CAD build for the part. Positions are in the model's coordinates, mm. A direction names the side the tool comes from. Round coordinates to 2 decimals unless told otherwise and drop trailing zeros. Answer as a JSON object with one key per item and string values.
```python
from build123d import *

# Parameters (mm, degrees)
F0_W          = 137.9242166877
F0_H          = 54.1928205639
F1_DEPTH      = 109.22
F1_TAPER      = -3
F2_T          = -5.08
F3_R          = 15.9007904293
F4_DEPTH      = 38.1
F4_TAPER      = -1
F5_T          = 2.54
F5_T3_DEPTH   = 109.5056366308
F5_T5_DEPTH   = 133.3627366899
F5_T7_DEPTH   = 109.5056366308
F5_T9_DEPTH   = 49.6313405661
F5_T11_DEPTH  = 109.5056366308
F5_T13_DEPTH  = 109.5056366308
F6_R          = 10.3601813923
F7_DEPTH      = 28.194
F7_DEPTH_BACK = 25.4


# Not quite as in the source:
# - a shell that OpenCascade refuses in one call is made with other operations: the cavity is built on its own and cut out


with BuildPart() as f1:
    # F0 (on Top) → F1 (new body)
    with BuildSketch(Plane.XY):
        with Locations((1.1629350483, -2.7910461649)):
            Rectangle(F0_W, F0_H)
    extrude(amount=F1_DEPTH, taper=F1_TAPER)

    # F2
    f2_openings = [f1.faces().sort_by_distance(p)[0] for p in [
        (1.162935, -2.791046, 109.22),
    ]]
    offset(amount=F2_T, openings=f2_openings)

    # F3 (on face) → F4 (join)
    with BuildSketch(Plane(origin=(0, -29.8055931401, -1.5620449467), x_dir=(1, 0, 0), z_dir=(0, -0.9986295348, -0.0523359562))):
        with Locations((0, 55.6432977319)):
            Circle(F3_R)
    extrude(amount=F4_DEPTH, taper=F4_TAPER)

    # F5: shell of thickness 2.54, made by hand


with BuildPart() as f5_core1:
    # F5_t2: copy of F1
    add(f1.part)

    # the walls: a layer under each face that stays
    f5_faces = [f5_core1.faces().sort_by_distance(p)[0] for p in [
        (1.1629350483, 27.1673529437, 54.61),
        (1.1629350483, -2.7910461649, 0),
        (-70.6611621221, -2.7910461649, 54.61),
        (72.0872036906, 9.6217245219, 109.22),
        (72.9870322188, -2.7910461649, 54.61),
        (-45.4478013646, -30.8414527224, 18.2033333333),
        (1.1629350483, -27.7955895152, 57.15),
        (68.0331764605, -2.7910461649, 57.15),
        (1.1629350483, 22.2134971854, 57.15),
        (-65.7073063639, -2.7910461649, 57.15),
        (-16.2333094162, -51.7416309725, 53.0079956131),
        (1.1629350483, -2.7910461649, 5.08),
    ]]
    thicken(f5_faces, amount=-F5_T, mode=Mode.SUBTRACT)

    # F5_s4 → F5_t3 (cut)
    with BuildSketch(Plane(origin=(-0.3725269372, -0.3725269372, 7.1082374087), x_dir=(0.7071067812, -0.7071067812, 0), z_dir=(-0.0522644277, -0.0522644277, 0.9972646886))):
        Polygon((-26.8076320701, -61.6755807303), (-25.0140422716, -63.5100601973), (-26.8076320701, -65.2987439692), (-28.6012218685, -63.5100601973), align=None)
    extrude(amount=F5_T3_DEPTH, mode=Mode.SUBTRACT)

    # F5_s6 → F5_t5 (cut)
    with BuildSketch(Plane.YZ.offset(-65.5184332966)):
        Polygon((-25.0413512578, 5.1067293333), (-27.6032354663, 4.9470666711), (-27.4770864474, 2.54), (-25.066716448, 2.54), align=None)
        Polygon((19.4592589279, 5.1067293333), (22.0211431364, 4.9470666711), (21.8949941176, 2.54), (19.4846241181, 2.54), align=None)
    extrude(amount=F5_T5_DEPTH, mode=Mode.SUBTRACT)

    # F5_s8 → F5_t7 (cut)
    with BuildSketch(Plane(origin=(0.3788802151, -0.3788802151, 7.229465173), x_dir=(0.7071067812, 0.7071067812, 0), z_dir=(0.0522644277, -0.0522644277, 0.9972646886))):
        Polygon((28.4522705876, -63.3157206494), (26.6586807892, -65.1502001164), (28.4522705876, -66.9388838882), (30.245860386, -65.1502001164), align=None)
    extrude(amount=F5_T7_DEPTH, mode=Mode.SUBTRACT)

    # F5_s10 → F5_t9 (cut)
    with BuildSketch(Plane.XZ.offset(-22.0246241181)):
        Polygon((65.2789382031, 5.1067293333), (67.8408224115, 4.9470666711), (67.7146733927, 2.54), (65.3043033933, 2.54), align=None)
        Polygon((-62.9530681064, 5.1067293333), (-65.5149523149, 4.9470666711), (-65.388803296, 2.54), (-62.9784332966, 2.54), align=None)
    extrude(amount=F5_T9_DEPTH, mode=Mode.SUBTRACT)

    # F5_s12 → F5_t11 (cut)
    with BuildSketch(Plane(origin=(6.0868817641, 6.0868817641, 116.1446229433), x_dir=(0.7071067812, -0.7071067812, 0), z_dir=(-0.0522644277, -0.0522644277, -0.9972646886))):
        Polygon((32.3994059273, -59.3793819539), (34.1929957257, -61.2138614209), (32.3994059273, -63.0025451928), (30.6058161288, -61.2138614209), align=None)
    extrude(amount=F5_T11_DEPTH, mode=Mode.SUBTRACT)

    # F5_s14 → F5_t13 (cut)
    with BuildSketch(Plane(origin=(-0.357279059, 0.357279059, 6.8172905608), x_dir=(-0.7071067812, -0.7071067812, 0), z_dir=(-0.0522644277, 0.0522644277, 0.9972646886))):
        Polygon((30.7547674097, -57.7392420349), (28.9611776113, -59.5737215018), (30.7547674097, -61.3624052737), (32.5483572082, -59.5737215018), align=None)
    extrude(amount=F5_T13_DEPTH, mode=Mode.SUBTRACT)

    # F5_s15 → F5_t16 (revolve, cut)
    with BuildSketch(Plane(origin=(0, -2.9121451953, 55.5670405262), x_dir=(1, 0, 0), z_dir=(0, 0.0523359562, -0.9986295348))):
        Polygon((15.9261865608, 29.8714534354), (15.9007904293, 27.3064967266), (13.3160676512, 27.3064967266), (13.3611772836, 29.8908258389), align=None)
    revolve(axis=Axis((0, -32.7177383354, 54.0049955795), (0, -0.9986295348, -0.0523359562)), mode=Mode.SUBTRACT)


with BuildPart() as f1_1:
    add(f1.part)

    # what is left inside the walls is the cavity
    f5_cavity = [f5_core1.part.solids().sort_by_distance(p)[0] for p in [
        (-13.557203, -45.430288, 53.338759),
    ]]
    add(f5_cavity, mode=Mode.SUBTRACT)

    # F6 (on face) → F7 (cut, two sides)
    with BuildSketch(Plane(origin=(0, -29.8055931401, -1.5620449467), x_dir=(1, 0, 0), z_dir=(0, -0.9986295348, -0.0523359562))) as f7_sk:
        with Locations((0, 55.7023957372)):
            Circle(F6_R)
    extrude(amount=-F7_DEPTH, mode=Mode.SUBTRACT)
    extrude(f7_sk.sketch, amount=F7_DEPTH_BACK, mode=Mode.SUBTRACT)


solid = f1_1.part
```
Item 1: Drop flat-ended pins along their axis: pin 1 Ø10 at (x, y) = (-44.5, 19.5) entering from -Z; pin 2 Ø1.5 at (y, z) = (-17.5, 12) entering from +X; pin 3 Ø3 at (y, z) = (-14.5, 66) entering from +X; pin 4 Ø10 at (x, z) = (25, 29) entering from +Y. Give the stop position or say it passes through.
Worked answers:
{"pin 1": "stops at z = 0", "pin 2": "stops at x = 70.79", "pin 3": "stops at x = 73.66", "pin 4": "stops at y = 26.09"}
Item 2: Two-plate mould, pull along Y, no slides. Class faces 1 (the conical face through (8.729, -52.725, 66.667)), 2 (the flat face through (-12.348, -71.155, 59.441)), 3 (the flat face through (0, -3, 0)): released by +Y, released by -Y, zero draft, split by the parting line, or undercut.
Worked answers:
{"face 1": "undercut", "face 2": "released by -Y", "face 3": "zero draft"}
Item 3: Wall check: line 1 along Z through (x, y) = (-28, 5.5); line 2 along Y through (x, z) = (-61.5, 9); line 3 along X through (y, z) = (13, 58.5). Give the ranges that are in metal, low to high. Write a range as [from, to].
Worked answers:
{"line 1": "z = [0, 5.08]", "line 2": "y = [-30.36, -25.27], [19.69, 24.78]", "line 3": "x = [-70.87, -65.78], [68.1, 73.19]"}
Item 4: 3-axis set-ups, long thin cutter, end or side, ignore diameter. For faces 4 (the flat face through (-65.746, -2.403, 57.879)), 5 (the flat face through (1, 27, 109.22)): which of +Z, -Z, +X, -X, +Y, -Y reach the whole face in a straight line?
Worked answers:
{"face 4": "+Z", "face 5": "+Z, +X, -X, +Y, -Y"}
